Drawing for the job (mm, zero at the part's lowest x, y, z). Coordinates: 2 decimals unless noted, no trailing zeros. Write each loop counter-clockwise with the first axis right and the second up, starting at its lowest first coordinate (ties: lowest second). Pieces come first, ordered by that corner, then holes. Notation, with made-up numbers: M -10,-7.5 L 31,-7.5 A21 cw 31,16.5 Z; hole C 80.25,61 d4. An arc over 180 degrees is marked long. Use a Markdown table: item, result. Add a question column.
Q1. Wall check: L1, parallel to X at y = 3.75, z = 82.55 (1 decimal); L2, parallel to X at y = 2, z = 73 (1 decimal); L3, parallel to Z at x = 39, y = 4.5. Give the ranges that are in metal, low to high. Write a range as from..to.
Q2. Pin check, flat tip, straight feed: pin 1 Ø3.5 at (x, z) = (25.12, 64.36) entering from +Y. Stop position of the tip, or through.
Q3. Slice it at A-A on z = 82.55. Count the separate pieces of the cut face and the enclosed holes in it, then the cut area to 3 significant figures.
Q4. Slice it at B-B on x = 103. Write the cut outline in (y, z).
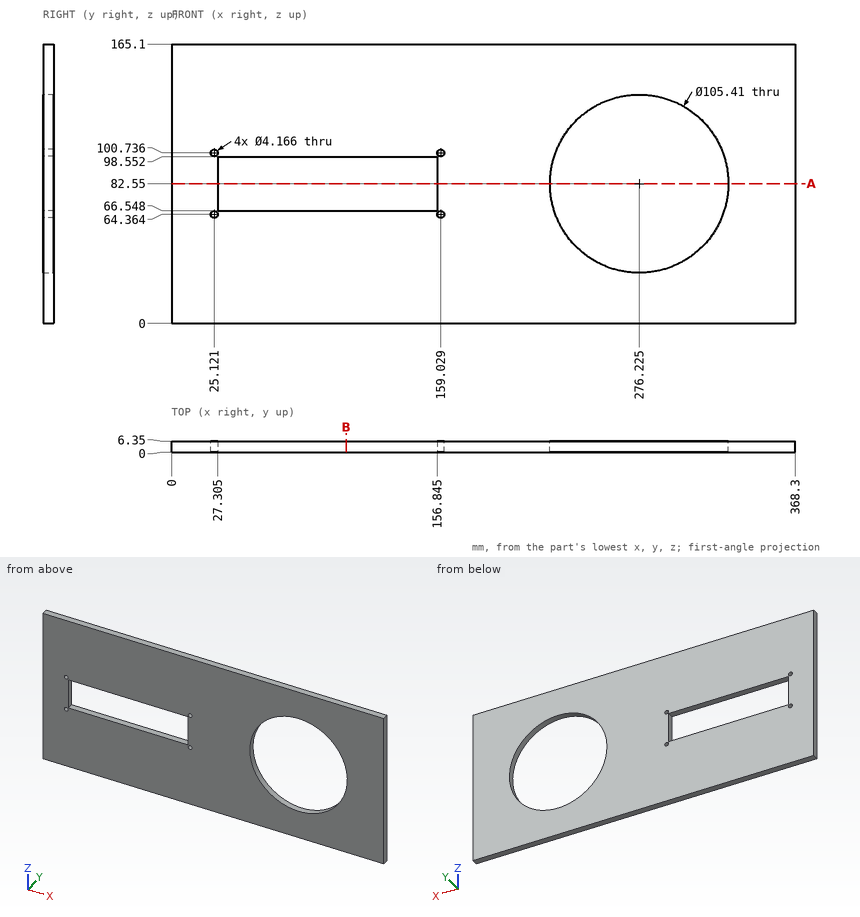
Recorded:
| question | item | result |
|---|---|---|
| 1 | L1 | 0..27.3, 156.8..223.5, 328.9..368.3 |
| 1 | L2 | 0..27.3, 156.8..224.4, 328.1..368.3 |
| 1 | L3 | 0..66.55, 98.55..165.1 |
| 2 | pin 1 | through |
| 3 | separate pieces | 3 |
| 3 | enclosed holes | 0 |
| 3 | area | 847 mm² |
| 4 | outline | M 0,0 L 6.35,0 L 6.35,66.55 L 0,66.55 Z; M 0,98.55 L 6.35,98.55 L 6.35,165.1 L 0,165.1 Z |
